Could you check a few things on this model? Use its own coordinates, in mm. A direction names the side the tool comes from. Give positions to 0.01 mm unless a question says otherwise; leave off trailing zeros. Write each loop counter-clockwise with the first axis right and the second up, starting at its lowest first coordinate (ties: lowest second). Pieces come first, ordered by that corner, then holes. Notation, with made-up numbers: M 1.25,-18.5 L 14.25,-18.5 A28 ccw 14.25,19.5 Z; hole C 12,85 d11. An arc over 180 degrees is marked long. Answer as a JSON object with one key per item and string values. Group by question number.
```python
from build123d import *

# Parameters (mm, degrees)
SKETCH1_W                                = 63.5
SKETCH1_H                                = 95.25
BOSS_EXTRUDE1_DEPTH                      = 8.89
CUT_EXTRUDE1_DEPTH                       = 3.81
CUT_EXTRUDE2_DEPTH                       = 1.905
MIRROR2_AT_THE_SECOND_PLANE_COPY_1_DEPTH = 1.905
FILLET1_R                                = 15.24


with BuildPart() as part:
    # Sketch1 → Boss-Extrude1 (new body)
    with BuildSketch(Plane.XY):
        Rectangle(SKETCH1_W, SKETCH1_H)
    extrude(amount=-BOSS_EXTRUDE1_DEPTH)

    # Sketch4 → Cut-Extrude1 (cut)
    with BuildSketch(Plane.XY):
        with BuildLine():
            Line((-15.321546842, -43.089479105), (14.859998977, -43.1))
            ThreePointArc((14.859998977, -43.1), (24.052387544, -39.292388268), (27.86, -30.1))
            Line((27.86, -30.1), (27.86, 29.848016994))
            ThreePointArc((27.86, 29.848016994), (24.142757308, 39.204832311), (14.858601027, 43.099999609))
            Line((14.858601027, 43.099999609), (-15.322946088, 43.094305911))
            ThreePointArc((-15.322946088, 43.094305911), (-24.214524383, 39.131012084), (-27.86, 30.104475598))
            Line((-27.86, 30.104475598), (-27.86, -30.1))
            ThreePointArc((-27.86, -30.1), (-24.214594541, -39.127455295), (-15.321546842, -43.089479105))
        make_face()
    extrude(amount=-CUT_EXTRUDE1_DEPTH, mode=Mode.SUBTRACT)

    # Sketch8 → Revolve1 (revolve)
    with BuildSketch(Plane.ZX.offset(33.02), mode=Mode.PRIVATE) as revolve1_sk:
        Polygon((-3.81, -17.78), (-2.921, -17.78), (-0.635, -17.78), (-0.635, -16.51), (-2.54, -16.764), (-3.81, -16.51), align=None)
    revolve1 = revolve(revolve1_sk.sketch.rotate(Axis((-17.78, 33.02, -3.81), (0, 0, 1)), 180), axis=Axis((-17.78, 33.02, -3.81), (0, 0, 1)))

    # Sketch9 → Revolve2 (revolve)
    with BuildSketch(Plane.ZX.offset(33.02), mode=Mode.PRIVATE) as revolve2_sk:
        Polygon((-3.81, 17.78), (-2.54, 17.78), (-0.635, 17.78), (-0.635, 19.05), (-2.54, 18.796), (-3.81, 19.05), align=None)
    revolve2 = revolve(revolve2_sk.sketch.rotate(Axis((17.78, 33.02, -3.81), (0, 0, 1)), 180), axis=Axis((17.78, 33.02, -3.81), (0, 0, 1)))

    # Mirror1: Revolve1, Revolve2 across plane
    add(revolve1.mirror(Plane.ZX))
    add(revolve2.mirror(Plane.ZX))

    # Sketch10 → Cut-Extrude2 (cut)
    with BuildSketch(Plane.XY.offset(-0.635)):
        with BuildLine():
            Line((-17.53, 31.774849407), (-17.53, 34.265150593))
            ThreePointArc((-17.53, 34.265150593), (-17.78, 34.29), (-18.03, 34.265150593))
            Line((-18.03, 34.265150593), (-18.03, 31.774849407))
            ThreePointArc((-18.03, 31.774849407), (-17.78, 31.75), (-17.53, 31.774849407))
        make_face()
    cut_extrude2 = extrude(amount=-CUT_EXTRUDE2_DEPTH, mode=Mode.SUBTRACT)

    # Mirror2: Cut-Extrude2 across plane
    add(cut_extrude2.mirror(Plane.ZX), mode=Mode.SUBTRACT)

    # Mirror2 at the second plane: Cut-Extrude2 across plane
    add(cut_extrude2.mirror(Plane(origin=(0, 0, 0), x_dir=(0, 0, 1), z_dir=(1, 0, 0))), mode=Mode.SUBTRACT)

    # Mirror2 at the second plane copy 1 sketc → Mirror2 at the second plane copy 1 (cut)
    with BuildSketch(Plane(origin=(0, 0, -0.635), x_dir=(-1, 0, 0), z_dir=(0, 0, 1))):
        with BuildLine():
            Line((-17.53, 31.774849407), (-17.53, 34.265150593))
            ThreePointArc((-17.53, 34.265150593), (-17.78, 34.29), (-18.03, 34.265150593))
            Line((-18.03, 34.265150593), (-18.03, 31.774849407))
            ThreePointArc((-18.03, 31.774849407), (-17.78, 31.75), (-17.53, 31.774849407))
        make_face()
    extrude(amount=-MIRROR2_AT_THE_SECOND_PLANE_COPY_1_DEPTH, mode=Mode.SUBTRACT)

    # Fillet1
    fillet1_edges = [part.edges().sort_by_distance(p)[0] for p in [
        (31.75, -47.625, -4.445),
        (-31.75, -47.625, -4.445),
        (-31.75, 47.625, -4.445),
        (31.75, 47.625, -4.445),
    ]]
    fillet(fillet1_edges, radius=FILLET1_R)


solid = part.part
```
1) We'd pull the mould along X, two halves only. Please class faces 1 (the flat face through (28.1, 3.8, 0)), 2 (the conical face through (-18.8, 33.4, -2.9)), 3 (the flat face through (31.75, 0, -4)): released by +X, released by -X, zero draft, split by the parting line, or undercut.
2) I'm going to push flat-ended pins straight in: pin 1 (5 mm diameter, centred on x = -20, y = -10.5, fed in from +Z); pin 2 (2 mm diameter, centred on y = -33, z = -2, fed in from -X); pin 3 (2 mm diameter, centred on x = 20, z = -7.5, fed in from -Y); pin 4 (1.5 mm diameter, centred on y = -33.5, z = -1, fed in from +X). Where does each tip first touch, or does it pass through?
3) If we section it at B-B, the plane x = 0.5: List the corners of the cut face in (y, z) for me (3 decimals), plus the area to 3 significant figures.
4) For faces 4 (the flat face through (-31.75, 0, -4)), 5 (the conical face through (18.92, -33, -1.6)), 6 (the flat face through (0, 1, -3.81)), which set-ups out of +Z, -Z, +X, -X, +Y, -Y let a thin tool reach every point of the face, with its end or its side?
5) If we section it at A-A, the plane z = -5.5: List the corners of the cut face in (x, y) for me (3 decimals), plus the area to 3 significant figures.
6) Please list where these lines run through material, in increasing order: line 1 along X through (y, z) = (-19, -0.5); line 2 along Y through (x, z) = (-15.5, -1) (3 decimals); line 3 along Z through (x, y) = (5.5, 35.5). Write a range as from..to.
Taken from the geometry:
{
 "1": {"face 1": "zero draft", "face 2": "undercut", "face 3": "released by +X"},
 "2": {"pin 1": "z = -3.81", "pin 2": "x = -31.75", "pin 3": "y = -47.42", "pin 4": "x = 31.75"},
 "3": {"outline": "M -47.625,-8.89 L 47.625,-8.89 L 47.625,0 L 43.097,0 L 43.097,-3.81 L -43.095,-3.81 L -43.095,0 L -47.625,0 Z", "area": "518 mm²"},
 "4": {"face 4": "+Z, -Z, -X, +Y, -Y", "face 5": "none", "face 6": "+Z"},
 "5": {"outline": "M -31.75,-32.385 A15.24 ccw -16.51,-47.625 L 16.51,-47.625 A15.24 ccw 31.75,-32.385 L 31.75,32.385 A15.24 ccw 16.51,47.625 L -16.51,47.625 A15.24 ccw -31.75,32.385 Z", "area": "5,850 mm²"},
 "6": {"line 1": "-31.75..-27.86, 27.86..31.75", "line 2": "-47.625..-43.082, 43.087..47.625", "line 3": "-8.89..-3.81"}
}
